from build123d import *

# Parameters (mm, degrees)
SKETCH1_W           = 82.55
SKETCH1_H           = 41.275
SKETCH1_R           = 12.1285
BOSS_EXTRUDE1_DEPTH = 15.875
SKETCH2_R           = 13.97
SKETCH2_R_2         = 10.795
BOSS_EXTRUDE2_DEPTH = 82.55


with BuildPart() as part:
    # Sketch1 → Boss-Extrude1 (new body)
    with BuildSketch(Plane(origin=(0, 0, 0), x_dir=(1, 0, 0), z_dir=(0, 1, 0))):
        Rectangle(SKETCH1_W, SKETCH1_H)
        with Locations(Location((17.78, 0, 0), (0, 0, 270))):
            Circle(SKETCH1_R, mode=Mode.SUBTRACT)
        with Locations(Location((-17.78, 0, 0), (0, 0, 90))):
            Circle(SKETCH1_R, mode=Mode.SUBTRACT)
    extrude(amount=BOSS_EXTRUDE1_DEPTH)

    # Sketch2 → Boss-Extrude2 (add)
    with BuildSketch(Plane(origin=(41.275, 0, 0), x_dir=(0, 0, -1), z_dir=(1, 0, 0))):
        with Locations((32.133455539, 7.9375)):
            Circle(SKETCH2_R)
        with Locations((32.133455539, 7.9375)):
            Circle(SKETCH2_R_2, mode=Mode.SUBTRACT)
    extrude(amount=-BOSS_EXTRUDE2_DEPTH)


solid = part.part
Design review of the part built by this model. Coordinates are the model's own, in mm. A direction names the side the tool comes from. Round coordinates to 2 decimals unless told otherwise and drop trailing zeros. Write each loop counter-clockwise with the first axis right and the second up, starting at its lowest first coordinate (ties: lowest second). Pieces come first, ordered by that corner, then holes. Notation, with made-up numbers: M 71.25,25.25 L 90.25,25.25 A8 ccw 90.25,29.25 Z; hole C 89.5,-39.5 d8. An arc over 180 degrees is marked long. One line per item, written item: value. Start each with the question number.
1. For faces 4 (the face through (-1, 0, 0)), 5 (the face through (-1, 8, 20.638)), list the 3-axis set-ups (+Z, -Z, +X, -X, +Y, -Y) from which the entire face can be reached by the end or side of a thin tool; tool diameter is ignored.
2. Clearance check with flat-ended pins moving along their axes: P1, Ø2, axis at x = 12, z = -31.5, coming from the +Y side; P2, Ø12.5, axis at x = 1.5, z = 1.5, coming from the +Y side (3 decimals); P3, Ø6, axis at x = -30.5, y = -1, coming from the -Z side; P4, Ø12.5, axis at x = -1.5, z = 1.5, coming from the -Y side. State where each tip first meets the part, or that it passes through.
3. Take a section at A-A on z = 0. State the section outline as (x, y) points (1 decimal), then the cut area to 3 significant figures.
4. Draft analysis for pull direction Y (two halves, no side actions). For faces 1 (the face through (0.578, 1.369, -23.567)), 2 (the face through (-1, 15.875, 0)), 3 (the face through (-13.13, 7.83, -11.2)), state which applies: pulls with the +Y half, pulls with the -Y half, needs draft (parallel to the pull), parting line crosses it, or undercut.
5. Take a section at C-C on y = 1.25. State the section outline as (x, z) points (1 decimal).
6. Take a section at D-D on x = -17.78. State the section outline as (y, z) points (1 decimal), then the cut area to 3 significant figures.
7. Take a section at B-B on x = 10. State the section outline as (y, z) points (1 decimal).
8. To check wall thickness, follow probe 1 along X at (y, z) = (7.5, 0) (1 decimal); probe 2 along Z at (x, y) = (7.5, 3); probe 3 along Z at (x, y) = (-13, 13). State the ranges of each line that lie inside material, in increasing order. Write a range as from..to.
Computed:
1. face 4: +Z, +X, -X, -Y
1. face 5: +Z, +X, -X, +Y, -Y
2. P1: stops at y = 21.91
2. P2: stops at y = 15.875
2. P3: stops at z = -44.78
2. P4: stops at y = 0
3. outline: M -41.3,0 L -29.9,0 L -29.9,15.9 L -41.3,15.9 Z; M -5.7,0 L 5.7,0 L 5.7,15.9 L -5.7,15.9 Z; M 29.9,0 L 41.3,0 L 41.3,15.9 L 29.9,15.9 Z
3. area: 540 mm²
4. face 1: undercut
4. face 2: pulls with the +Y half
4. face 3: needs draft
5. outline: M -41.3,-44.4 L 41.3,-44.4 L 41.3,-40.6 L -41.3,-40.6 Z; M -41.3,-23.7 L 41.3,-23.7 L 41.3,20.6 L -41.3,20.6 Z; hole C -17.8,0 d24.3; hole C 17.8,0 d24.3
6. outline: M 0,-20.6 A14 ccw long 15.9,-20.6 L 15.9,-12.1 L 0,-12.1 Z; M 0,12.1 L 15.9,12.1 L 15.9,20.6 L 0,20.6 Z; hole C 7.9,-32.1 d21.6
6. area: 490 mm²
7. outline: M 0,-20.6 A14 ccw long 15.9,-20.6 L 15.9,-9.3 L 0,-9.3 Z; M 0,9.3 L 15.9,9.3 L 15.9,20.6 L 0,20.6 Z; hole C 7.9,-32.1 d21.6
8. probe 1: x = -41.3..-29.9, -5.7..5.7, 29.9..41.3
8. probe 2: z = -45.2..-41.73, -22.53..-6.44, 6.44..20.64
8. probe 3: z = -45.15..-41.67, -22.6..-11.15, 11.15..20.64
